Input: part model. Units: mm. Frame: model coordinates. Round coordinates to 2 decimals unless told otherwise and drop trailing zeros. Write each loop counter-clockwise with the first axis right and the second up, starting at its lowest first coordinate (ties: lowest second). Pieces come first, ordered by that corner, then holes. Notation, with made-up numbers: (46, -14) -> (72, -14) arc R21 ccw to (72, 6) -> close; hole circle Ø3 at (-20.5, 34). An arc over 180 degrees is marked (long way). Use CSV: the item, a comma, the result in double quotes.
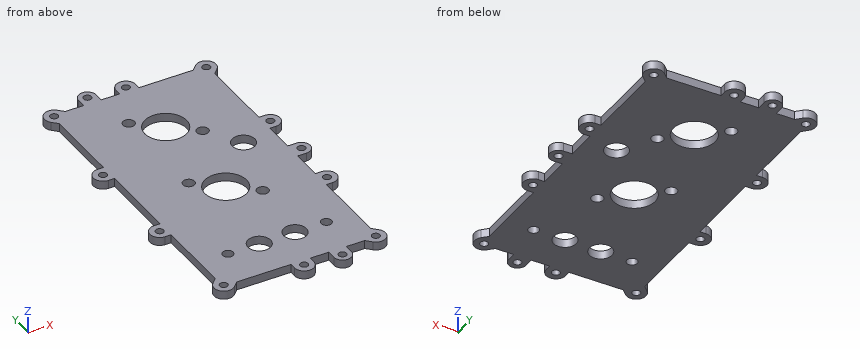
```python
from build123d import *

# Parameters (mm, degrees)
BOSS_EXTRUDE1_DEPTH  = 4.7625
M4_CLEARANCE_HOLE1_D = 4.5
SKETCH4_R            = 3.3
SKETCH4_R_2          = 2.9765625
SKETCH4_R_3          = 6.445
SKETCH4_R_4          = 11.9
CUT_EXTRUDE1_DEPTH   = 4.7625
BOSS_EXTRUDE3_DEPTH  = 4.7625
M4_CLEARANCE_HOLE2_D = 4.5


with BuildPart() as part:
    # Sketch1 → Boss-Extrude1 (new body)
    with BuildSketch(Plane.XY):
        with BuildLine():
            Line((50.349976536, 7.779015878), (19.528151129, 7.779015878))
            Line((19.528151129, 7.779015878), (16.547693582, 10.759473425))
            ThreePointArc((16.547693582, 10.759473425), (8.769518989, 10.759473425), (8.769518989, 2.981298831))
            Line((8.769518989, 2.981298831), (11.749976536, 0.000841285))
            Line((11.749976536, 0.000841285), (11.749976536, -43.901984122))
            Line((11.749976536, -43.901984122), (8.340276536, -43.901984122))
            ThreePointArc((8.340276536, -43.901984122), (2.840276536, -49.401984122), (8.340276536, -54.901984122))
            Line((8.340276536, -54.901984122), (11.749976536, -54.901984122))
            Line((11.749976536, -54.901984122), (11.749976536, -100.289984122))
            Line((11.749976536, -100.289984122), (8.340276536, -100.289984122))
            ThreePointArc((8.340276536, -100.289984122), (2.840276536, -105.789984122), (8.340276536, -111.289984122))
            Line((8.340276536, -111.289984122), (11.749976536, -111.289984122))
            Line((11.749976536, -111.289984122), (11.749976536, -155.192809529))
            Line((11.749976536, -155.192809529), (8.769518989, -158.173267075))
            ThreePointArc((8.769518989, -158.173267075), (8.769518989, -165.951441668), (16.547693582, -165.951441668))
            Line((16.547693582, -165.951441668), (19.528151129, -162.970984122))
            Line((19.528151129, -162.970984122), (50.349976536, -162.970984122))
            Line((50.349976536, -162.970984122), (50.349976536, -166.380684122))
            ThreePointArc((50.349976536, -166.380684122), (55.849976536, -171.880684122), (61.349976536, -166.380684122))
            Line((61.349976536, -166.380684122), (61.349976536, -162.970984122))
            Line((61.349976536, -162.970984122), (92.171801943, -162.970984122))
            Line((92.171801943, -162.970984122), (95.152259489, -165.951441668))
            ThreePointArc((95.152259489, -165.951441668), (102.930434082, -165.951441668), (102.930434082, -158.173267075))
            Line((102.930434082, -158.173267075), (99.949976536, -155.192809529))
            Line((99.949976536, -155.192809529), (99.949976536, -111.289984122))
            Line((99.949976536, -111.289984122), (103.359676536, -111.289984122))
            ThreePointArc((103.359676536, -111.289984122), (108.859676536, -105.789984122), (103.359676536, -100.289984122))
            Line((103.359676536, -100.289984122), (99.949976536, -100.289984122))
            Line((99.949976536, -100.289984122), (99.949976536, -54.901984122))
            Line((99.949976536, -54.901984122), (103.359676536, -54.901984122))
            ThreePointArc((103.359676536, -54.901984122), (108.859676536, -49.401984122), (103.359676536, -43.901984122))
            Line((103.359676536, -43.901984122), (99.949976536, -43.901984122))
            Line((99.949976536, -43.901984122), (99.949976536, 0.000841285))
            Line((99.949976536, 0.000841285), (102.930434082, 2.981298831))
            ThreePointArc((102.930434082, 2.981298831), (102.930434082, 10.759473425), (95.152259489, 10.759473425))
            Line((95.152259489, 10.759473425), (92.171801943, 7.779015878))
            Line((92.171801943, 7.779015878), (61.349976536, 7.779015878))
            Line((61.349976536, 7.779015878), (61.349976536, 11.188715878))
            ThreePointArc((61.349976536, 11.188715878), (55.849976536, 16.688715878), (50.349976536, 11.188715878))
            Line((50.349976536, 11.188715878), (50.349976536, 7.779015878))
        make_face()
    extrude(amount=-BOSS_EXTRUDE1_DEPTH)

    # M4 Clearance Hole1 (through all)
    with Locations(Plane(origin=(0, 0, -4.7625), x_dir=(-1, 0, 0), z_dir=(0, 0, -1))):
        with Locations((-12.658606286, -162.062354372), (-55.849976536, -166.380684122), (-99.041346785, -162.062354372), (-103.359676536, -105.789984122), (-103.359676536, -49.401984122), (-99.041346785, 6.870386128), (-12.658606286, 6.870386128), (-8.340276536, -49.401984122), (-8.340276536, -105.789984122), (-55.849976536, 11.188715878)):
            Hole(M4_CLEARANCE_HOLE1_D / 2)

    # Sketch4 → Cut-Extrude1 (cut)
    with BuildSketch(Plane(origin=(0, 0, -4.7625), x_dir=(-1, 0, 0), z_dir=(0, 0, -1))):
        with Locations((-41.616084767, -16.665859852)):
            Circle(SKETCH4_R)
        with Locations((-70.083868304, -40.3002691)):
            Circle(SKETCH4_R)
        with Locations((-27.909976536, -139.508484122)):
            Circle(SKETCH4_R_2)
        with Locations((-41.616084767, -76.466699143)):
            Circle(SKETCH4_R)
        with Locations((-83.789976536, -139.508484122)):
            Circle(SKETCH4_R_2)
        with Locations((-70.083868304, -100.101108391)):
            Circle(SKETCH4_R)
        with Locations((-66.009976536, -139.508484122)):
            Circle(SKETCH4_R_3)
        with Locations((-82.519976536, -59.220984122)):
            Circle(SKETCH4_R_3)
        with Locations((-45.689976536, -139.508484122)):
            Circle(SKETCH4_R_3)
        with Locations((-55.849976536, -88.283903767)):
            Circle(SKETCH4_R_4)
        with Locations((-55.849976536, -28.483064476)):
            Circle(SKETCH4_R_4)
    extrude(amount=-CUT_EXTRUDE1_DEPTH, mode=Mode.SUBTRACT)

    # Sketch6 → Boss-Extrude3 (add)
    with BuildSketch(Plane.XY):
        with BuildLine():
            Line((39.939063832, 7.779015878), (39.939063832, 12.779015878))
            ThreePointArc((39.939063832, 12.779015878), (34.939063832, 17.779015878), (29.939063832, 12.779015878))
            Line((29.939063832, 12.779015878), (29.939063832, 7.779015878))
            Line((29.939063832, 7.779015878), (39.939063832, 7.779015878))
        make_face()
        with BuildLine():
            Line((81.760889239, -162.970984122), (71.760889239, -162.970984122))
            Line((71.760889239, -162.970984122), (71.760889239, -167.970984122))
            ThreePointArc((71.760889239, -167.970984122), (76.760889239, -172.970984122), (81.760889239, -167.970984122))
            Line((81.760889239, -167.970984122), (81.760889239, -162.970984122))
        make_face()
        with BuildLine():
            Line((99.949976536, -72.595984122), (99.949976536, -82.595984122))
            Line((99.949976536, -82.595984122), (104.949976536, -82.595984122))
            ThreePointArc((104.949976536, -82.595984122), (109.949976536, -77.595984122), (104.949976536, -72.595984122))
            Line((104.949976536, -72.595984122), (99.949976536, -72.595984122))
        make_face()
    extrude(amount=-BOSS_EXTRUDE3_DEPTH)

    # M4 Clearance Hole2 (through all)
    with Locations(Plane.XY):
        with Locations((34.939063832, 12.779015878), (104.949976536, -77.595984122), (76.760889239, -167.970984122)):
            Hole(M4_CLEARANCE_HOLE2_D / 2)


solid = part.part
```
Item 1: Section query A-A on y = -93. Return the cut outline in (x, z), plus the area to 3 significant figures.
Worked answers:
outline,"(11.75, -4.76) -> (44.92, -4.76) -> (44.92, 0) -> (11.75, 0) -> close; (66.78, -4.76) -> (99.95, -4.76) -> (99.95, 0) -> (66.78, 0) -> close"
area,"316 mm²"
Item 2: Section query B-B on x = 56. Return the cut outline in (y, z).
Worked answers:
outline,"(-171.88, -4.76) -> (-168.63, -4.76) -> (-168.63, 0) -> (-171.88, 0) -> close; (-164.14, -4.76) -> (-100.18, -4.76) -> (-100.18, 0) -> (-164.14, 0) -> close; (-76.38, -4.76) -> (-40.38, -4.76) -> (-40.38, 0) -> (-76.38, 0) -> close; (-16.58, -4.76) -> (8.94, -4.76) -> (8.94, 0) -> (-16.58, 0) -> close; (13.43, -4.76) -> (16.69, -4.76) -> (16.69, 0) -> (13.43, 0) -> close"
Item 3: Line query: line 1 (Y direction, x = 68.5, z = -2.5); line 2 (X direction, y = -137, z = -3.95); line 3 (Y direction, x = 86.5, z = -0.35). Output: solid intervals per line, ascending.
Worked answers:
line 1,"y = -162.97 to -145.45, -133.56 to -103, -97.21 to -43.2, -37.41 to 7.78"
line 2,"x = 11.75 to 26.31, 29.51 to 39.75, 51.63 to 60.07, 71.95 to 82.19, 85.39 to 99.95"
line 3,"y = -162.97 to -140.74, -138.28 to -64.29, -54.15 to 7.78"
Item 4: Section query D-D on y = -32. Return the cut outline in (x, z), plus the area to 3 significant figures.
Worked answers:
outline,"(11.75, -4.76) -> (44.48, -4.76) -> (44.48, 0) -> (11.75, 0) -> close; (67.22, -4.76) -> (99.95, -4.76) -> (99.95, 0) -> (67.22, 0) -> close"
area,"312 mm²"
Item 5: First-contact query: pin 1 Ø1.4 at (y, z) = (-94.5, -1.5) entering from +X; pin 2 Ø2.5 at (x, y) = (99.04, -162.06) entering from -Z; pin 3 Ø1.7 at (y, z) = (-164, -2.5) entering from -X; pin 4 Ø1.7 at (x, z) = (9.5, -1.5) entering from +Y. Flat tips, straight axial feed; report the tip coordinate or a pass-through.
Worked answers:
pin 1,"stops at x = 99.95"
pin 2,"passes through"
pin 3,"stops at x = 7.27"
pin 4,"stops at y = 11.86"
Item 6: Section query C-C on z = -2.2. Give the number of separate pieces and of enclosed holes in the cut face, plus the area to 3 significant figures.
Worked answers:
separate pieces,"1"
enclosed holes,"24"
area,"14,400 mm²"
